Could you check a few things on this model? Use its own coordinates, in mm. A direction names the side the tool comes from. Give positions to 0.01 mm unless a question says otherwise; leave off trailing zeros. Order: outer loops, then holes, each group sorted by start corner. A loop starts at its lowest first (then second) coordinate and runs counter-clockwise, first axis right, second up. Notation, with made-up numbers: M 3.5,-3.75 L 62.5,-3.75 A26 cw 62.5,12.25 Z; hole C -37,61 d10. An arc over 180 degrees is marked long. Use a Markdown table: item, result. Add a question column.
Item 1: If we mould it in two halves opening along Z, with no side actions, what happens to faces 1 (the face through (-2.86, -0.9, 0.75)), 2 (the face through (0, 0, 0)), 3 (the face through (-0.62, 2.78, 1.39))? For each: released by +Z, released by -Z, zero draft, split by the parting line, or undercut.
Item 2: If I drill on L1, parallel to X at y = -0.1, z = 3.75; L2, parallel to Y at x = -0.9, z = 8.5; L3, parallel to X at y = -1.2, z = 18.5, over which ranges is the centre line in solid material (lowest first)? Write a range as from..to.
Item 3: Suppose I cut it at A-A on z = 19. Write out the boundary of the cut face in (x, y), plus the area to 3 significant figures.
Item 4: I'm going to push flat-ended pins straight in: pin 1 Ø2 at (y, z) = (-2, 17) entering from -X; pin 2 Ø2 at (y, z) = (-1.5, 16) entering from +X. Where does each tip first touch, or does it pass through?
Item 5: For faces 4 (the face through (-2.86, -0.9, 10.38)), 5 (the face through (-2.262, -1.734, 19.594)), which set-ups out of +Z, -Z, +X, -X, +Y, -Y let a thin tool reach every point of the face, with its end or its side?
from build123d import *

# Parameters (mm, degrees)
SZKIC1_R                    = 3
DODANIE_WYCI_GNI_CIE1_DEPTH = 21
SFAZOWANIE1_SIZE            = 0.5
WYTNIJ_WYCI_GNI_CIE1_START  = -1.8
SZKIC2_R                    = 3
SZKIC2_R_2                  = 2.85
WYTNIJ_WYCI_GNI_CIE1_DEPTH  = 0.8
WYTNIJ_WYCI_GNI_CIE2_START  = -1
SZKIC3_R                    = 3
SZKIC3_R_2                  = 2.85
WYTNIJ_WYCI_GNI_CIE2_DEPTH  = 0.8


with BuildPart() as part:
    # Szkic1 → Dodanie-wyciągnięcie1 (new body)
    with BuildSketch(Plane.XY):
        with Locations(Location((0, 0, 0), (0, 0, 180))):
            Circle(SZKIC1_R)
    extrude(amount=DODANIE_WYCI_GNI_CIE1_DEPTH)

    # Sfazowanie1
    sfazowanie1_edges = [part.edges().sort_by_distance(p)[0] for p in [
        (3, 0, 0),
        (3, 0, 21),
    ]]
    chamfer(sfazowanie1_edges, length=SFAZOWANIE1_SIZE)

    # Szkic2 → Wytnij-wyciągnięcie1 (cut)
    with BuildSketch(Plane.XY.offset(21).offset(WYTNIJ_WYCI_GNI_CIE1_START)):
        with Locations(Location((0, 0, 0), (0, 0, 180))):
            Circle(SZKIC2_R)
        Circle(SZKIC2_R_2, mode=Mode.SUBTRACT)
    extrude(amount=WYTNIJ_WYCI_GNI_CIE1_DEPTH, mode=Mode.SUBTRACT)

    # Szkic3 → Wytnij-wyciągnięcie2 (cut)
    with BuildSketch(Plane(origin=(0, 0, 0), x_dir=(-1, 0, 0), z_dir=(0, 0, -1)).offset(WYTNIJ_WYCI_GNI_CIE2_START)):
        Circle(SZKIC3_R)
        with Locations(Location((0, 0, 0), (0, 0, 180))):
            Circle(SZKIC3_R_2, mode=Mode.SUBTRACT)
    extrude(amount=-WYTNIJ_WYCI_GNI_CIE2_DEPTH, mode=Mode.SUBTRACT)


solid = part.part
Findings below:
| question | item | result |
|---|---|---|
| 1 | face 1 | zero draft |
| 1 | face 2 | released by -Z |
| 1 | face 3 | undercut |
| 2 | L1 | x = -3..3 |
| 2 | L2 | y = -2.86..2.86 |
| 2 | L3 | x = -2.75..2.75 |
| 3 | outline | C 0,0 d6 |
| 3 | area | 28.3 mm^2 |
| 4 | pin 1 | stops at x = -2.83 |
| 4 | pin 2 | stops at x = 2.96 |
| 5 | face 4 | +Z, -Z |
| 5 | face 5 | none |
